from build123d import *

# Parameters (mm, degrees)
BLANKSKE_W              = 209
BLANKSKE_H              = 12.5
BLANK_DEPTH             = 14
TOOTHCUTILL_DEPTH       = 210.841011244
TOOTHCUTSIM_DEPTH       = 210.841011244
TEETHCUTS_COUNT         = 27
TEETHCUTS_PITCH         = 7.853981625
SKETCH8_W               = 209
SKETCH8_H               = 14
BOSS_EXTRUDE3_DEPTH     = 6.5
BOSS_EXTRUDE1_START     = -209
BOSS_EXTRUDE1_DEPTH     = 60
SKETCH4_R               = 1.75
CUT_EXTRUDE1_DEPTH      = 5
BOSS_EXTRUDE2_REACH     = 218.588
SKETCH6_W               = 26
SKETCH6_H               = 8
CUT_EXTRUDE2_DEPTH      = 214.593656273
CUT_EXTRUDE2_DEPTH_BACK = 214.593656273
SKETCH7_R               = 1.75
FILLET1_R               = 5
SKETCH9_W               = 14
SKETCH9_H               = 19
CUT_EXTRUDE3_DEPTH      = 40


with BuildPart() as part:
    # BlankSke → Blank (new body)
    with BuildSketch(Plane.XY):
        with Locations((104.5, 6.25)):
            Rectangle(BLANKSKE_W, BLANKSKE_H)
    extrude(amount=-BLANK_DEPTH)

    # TooCutSkeIll → ToothCutIll (cut, through all)
    with BuildSketch(Plane.XY):
        with BuildLine():
            Line((-3.110472484, 12.434202014), (-1.237006086, 7.28689539))
            ThreePointArc((-1.237006086, 7.28689539), (-1.007817354, 6.98821082), (-0.648758505, 6.875))
            Line((-0.648758505, 6.875), (0.648758505, 6.875))
            ThreePointArc((0.648758505, 6.875), (1.007817354, 6.98821082), (1.237006086, 7.28689539))
            Line((1.237006086, 7.28689539), (3.110472484, 12.434202014))
            ThreePointArc((3.110472484, 12.434202014), (3.147084102, 12.481915204), (3.204441746, 12.5))
            Line((3.204441746, 12.5), (3.204441746, 12.5254))
            Line((3.204441746, 12.5254), (-3.204441746, 12.5254))
            Line((-3.204441746, 12.5254), (-3.204441746, 12.5))
            ThreePointArc((-3.204441746, 12.5), (-3.147084102, 12.481915204), (-3.110472484, 12.434202014))
        make_face()
    extrude(amount=-TOOTHCUTILL_DEPTH, mode=Mode.SUBTRACT)

    # TooCutSkeSim → ToothCutSim (cut, through all)
    with BuildSketch(Plane.XY):
        Polygon((1.087088424, 6.875), (-1.087088424, 6.875), (-3.143665836, 12.5254), (3.143665836, 12.5254), align=None)
    toothcutsim = extrude(amount=-TOOTHCUTSIM_DEPTH, mode=Mode.SUBTRACT)

    # TeethCuts: ToothCutSim ×27
    with Locations(*[(i * TEETHCUTS_PITCH, 0, 0) for i in range(1, TEETHCUTS_COUNT)]):
        add(toothcutsim, mode=Mode.SUBTRACT)

    # Sketch8 → Boss-Extrude3 (add)
    with BuildSketch(Plane.XZ):
        with Locations((104.5, -7)):
            Rectangle(SKETCH8_W, SKETCH8_H)
    extrude(amount=BOSS_EXTRUDE3_DEPTH)

    # Sketch3 → Boss-Extrude1 (add)
    with BuildSketch(Plane(origin=(209, 0, 0), x_dir=(0, 0, -1), z_dir=(1, 0, 0)).offset(BOSS_EXTRUDE1_START)):
        Polygon((20.5, -6.5), (-13, -6.5), (-13, 51.5), (20.5, 51.5), (20.5, 46.5), (-8, 46.5), (-8, -1.5), (20.5, -1.5), align=None)
    extrude(amount=BOSS_EXTRUDE1_DEPTH)

    # Sketch4 → Cut-Extrude1 (cut)
    with BuildSketch(Plane.XY.offset(13)):
        with Locations((10, 40.5)):
            Circle(SKETCH4_R)
        with Locations((50, 40.5)):
            Circle(SKETCH4_R)
        with Locations((50, 4.5)):
            Circle(SKETCH4_R)
        with Locations((10, 4.5)):
            Circle(SKETCH4_R)
    extrude(amount=-CUT_EXTRUDE1_DEPTH, mode=Mode.SUBTRACT)

    # Boss-Extrude2: up to this face of the body (flat: up to its plane)
    boss_extrude2_end = Plane(part.part.faces().sort_by_distance((19.634954063, 12.5, -7))[0])
    # Sketch6 → Boss-Extrude2 (add, up to the picked face)
    with BuildSketch(Plane(origin=(0, -1.5, 0), x_dir=(1, 0, 0), z_dir=(0, 1, 0)), mode=Mode.PRIVATE) as boss_extrude2_sk1:
        with Locations((30, -4)):
            Rectangle(SKETCH6_W, SKETCH6_H)
    boss_extrude2_tool1 = split(extrude(boss_extrude2_sk1.sketch, amount=BOSS_EXTRUDE2_REACH, mode=Mode.PRIVATE), bisect_by=boss_extrude2_end, keep=Keep.BOTH, mode=Mode.PRIVATE)
    add(boss_extrude2_tool1.solids().sort_by(Axis((30, -1.5, 4), (0, 1, 0)))[0])

    # Sketch7 → Cut-Extrude2 (cut, two sides: drawn at the far end of the back side and taken through both)
    with BuildSketch(Plane(origin=(0, 12.5, 0), x_dir=(1, 0, 0), z_dir=(0, 1, 0)).offset(-CUT_EXTRUDE2_DEPTH_BACK)):
        with Locations(Location((20, 17, 0), (0, 0, 270))):
            Circle(SKETCH7_R)
        with Locations(Location((40, 17, 0), (0, 0, 270))):
            Circle(SKETCH7_R)
        with Locations(Location((40, -3, 0), (0, 0, 270))):
            Circle(SKETCH7_R)
        with Locations(Location((20, -3, 0), (0, 0, 270))):
            Circle(SKETCH7_R)
    extrude(amount=CUT_EXTRUDE2_DEPTH + CUT_EXTRUDE2_DEPTH_BACK, mode=Mode.SUBTRACT)

    # Fillet1
    fillet1_edges = [part.edges().sort_by_distance(p)[0] for p in [
        (30, -6.5, 13),
        (30, 51.5, 13),
    ]]
    fillet(fillet1_edges, radius=FILLET1_R)

    # Sketch9 → Cut-Extrude3 (cut)
    with BuildSketch(Plane(origin=(209, 0, 0), x_dir=(0, 0, -1), z_dir=(1, 0, 0))):
        with Locations((7, 3)):
            Rectangle(SKETCH9_W, SKETCH9_H)
    extrude(amount=-CUT_EXTRUDE3_DEPTH, mode=Mode.SUBTRACT)


solid = part.part
The listing builds one solid part. Answer for the finished solid, in the listing's coordinates (mm). A direction names the side the tool comes from. Round coordinates to 2 decimals unless told otherwise and drop trailing zeros. Write each loop counter-clockwise with the first axis right and the second up, starting at its lowest first coordinate (ties: lowest second). Pieces come first, ordered by that corner, then holes. Notation, with made-up numbers: M -24,35 L 30,35 A6 cw 30,43 Z; hole C 24.5,1.25 d2. An arc over 180 degrees is marked long. Write each question's results on one line, items separated by ' | '. Start each with the question number.
Item 1: Find section C-C on z = 3. Write down the section's boundary in (x, y).
Item 2: Straight lines are drawn through the part: probe 1 along X at (y, z) = (-4.45, -17); probe 2 along Z at (x, y) = (20, -3.5); probe 3 along X at (y, z) = (1.5, 3). For each, find the intervals that lie inside material, in ascending order.
Item 3: Find section A-A on y = 4.5. Write down the section's boundary in (x, z), and give its area (3 significant figures).
Item 4: Which of the six approach directions +Z, -Z, +X, -X, +Y, -Y give full straight-line access (tool end or side, diameter ignored) to faces 5 (the cylindrical face through (10.81, 2.95, 10.54)), 6 (the flat face through (135.643, 9.727, -6.902)), 7 (the flat face through (169, 3, -7)), 8 (the flat face through (49.25, 9.73, -6.9)), 9 (the cylindrical face through (21.735, 2.867, 2.772))?
Item 5: The mould has two halves that part along Z. Classify faces 1 (the flat face through (8, 4, 0)), 2 (the cylindrical face through (38.29, 48.96, 2.62)), 3 (the flat face through (100.005, 9.648, -6.902)), 4 (the flat face through (30, 49, -20.5)): +Z half, -Z half, draft (parallel to the pull), parting line (faces both ways), or undercut.
Item 6: Find section B-B on y = 40.5. Write down the section's boundary in (x, z).
Item 7: Given pin 1 Ø0.8 at (x, z) = (161.5, -4.5) entering from +Y; pin 2 Ø1 at (x, z) = (144.5, 1.5) entering from -Y; pin 3 Ø4 at (y, z) = (3.5, 3) entering from +X; pin 4 Ø3 at (x, y) = (24, 9) entering from -Z, each flat-ended and moving along its own axis, determine where each tip first touches the part or whether it passes through.
Item 8: Find section D-D on z = 10.5. Write down the section's boundary in (x, y), and give its area (3 significant figures).
Answer block:
1) outline: M 0,-6.5 L 18.25,-6.5 L 18.25,12.5 L 17,12.5 L 17,-1.5 L 0,-1.5 Z; M 0,46.5 L 18.25,46.5 L 18.25,51.5 L 0,51.5 Z; M 21.75,-6.5 L 38.25,-6.5 L 38.25,12.5 L 21.75,12.5 Z; M 21.75,46.5 L 38.25,46.5 L 38.25,51.5 L 21.75,51.5 Z; M 41.75,-6.5 L 60,-6.5 L 60,-1.5 L 43,-1.5 L 43,12.5 L 41.75,12.5 Z; M 41.75,46.5 L 60,46.5 L 60,51.5 L 41.75,51.5 Z
2) probe 1: x = 0 to 18.25, 21.75 to 38.25, 41.75 to 60 | probe 2: z = -20.5 to -18.75, -15.25 to 1.25, 4.75 to 12.58 | probe 3: x = 17 to 18.25, 21.75 to 38.25, 41.75 to 43
3) outline: M 0,-14 L 169,-14 L 169,0 L 43,0 L 43,8 L 48.25,8 L 48.25,13 L 11.75,13 L 11.75,8 L 17,8 L 17,0 L 0,0 Z; M 0,8 L 8.25,8 L 8.25,13 L 0,13 Z; M 51.75,8 L 60,8 L 60,13 L 51.75,13 Z; hole C 20,3 d3.5; hole C 40,3 d3.5 | area: 2,820 mm²
4) face 5: +Z | face 6: +Z, -Z, +Y | face 7: +Z, -Z, +X, +Y, -Y | face 8: -Z | face 9: +Y, -Y
5) face 1: undercut | face 2: undercut | face 3: draft | face 4: -Z half
6) outline: M 0,8 L 8.25,8 L 8.25,13 L 0,13 Z; M 11.75,8 L 48.25,8 L 48.25,13 L 11.75,13 Z; M 51.75,8 L 60,8 L 60,13 L 51.75,13 Z
7) pin 1: stops at y = 12.5 | pin 2: passes through | pin 3: stops at x = 43 | pin 4: stops at z = -14
8) outline: M 0,-5.83 L 60,-5.83 L 60,50.83 L 0,50.83 Z; hole C 10,4.5 d3.5; hole C 10,40.5 d3.5; hole C 50,4.5 d3.5; hole C 50,40.5 d3.5 | area: 3,360 mm²
